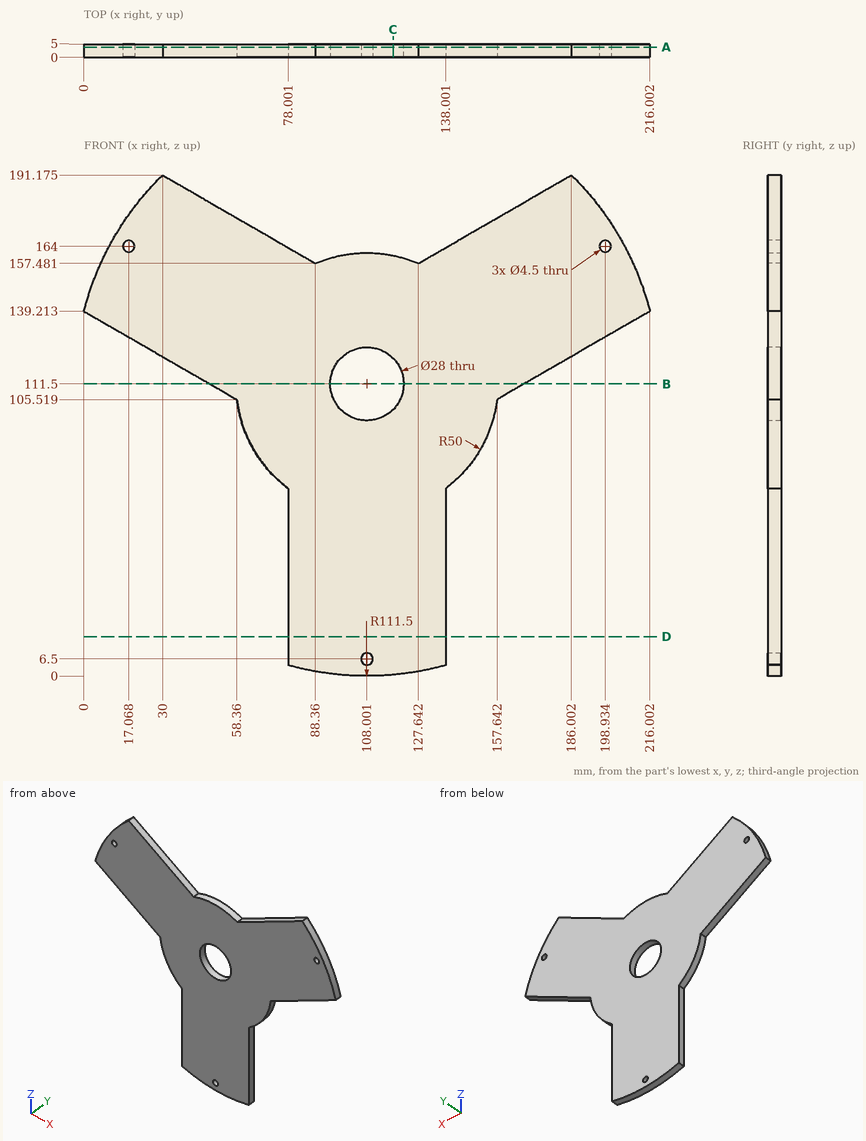
Geometry check sheet. Reference: drawing and pictorial views, mm from the part's lowest x, y, z. Round coordinates to 2 decimals unless told otherwise and drop trailing zeros. Loops run counter-clockwise (first coordinate to the right, second up) from the corner with the lowest first, then second, coordinate; pieces in that order, holes last. Notation, with made-up numbers: (36.25, -11.75) - (54.25, -11.75) arc R9 cw to (54.25, -1.75) - close; hole circle Ø9 at (-20.5, -28). An arc over 180 degrees is marked (long way). One line per question, with ' | ' between items. Start each with the question number.
1. Cross-section at D-D on z = 15. Record the cut outline in (x, y), then the cut area to 3 significant figures.
2. Cross-section at A-A on y = 3.85. State how many separate pieces and enclosed holes the cut face has, then the cut area to 3 significant figures.
3. Cross-section at B-B on z = 111.5. Record the cut outline in (x, y), then the cut area to 3 significant figures.
4. Scan lines: line 1 (X direction, y = 3.9, z = 164) (1 decimal); line 2 (X direction, y = 3.45, z = 52.5); line 3 (X direction, y = 3.6, z = 171) (1 decimal). Record each from-to range of solid material in increasing order. Write a range as [from, to].
5. Cross-section at C-C on x = 118. Record the cut outline in (y, z), then the cut area to 3 significant figures.
6. Depth check by flat-ended pin: pin 1 (2 mm diameter, centred on y = 1, z = 165, fed in from +X); pin 2 (3.5 mm diameter, centred on x = 17.07, z = 164, fed in from +Y); pin 3 (2 mm diameter, centred on y = 1.5, z = 27.5, fed in from -X). Enter the tip coordinate at first touch or a pass-through.
Taken from the geometry:
1) outline: (78, 0) - (138, 0) - (138, 5) - (78, 5) - close | area: 300 mm²
2) separate pieces: 1 | enclosed holes: 4 | area: 18,600 mm²
3) outline: (48, 0) - (94, 0) - (94, 5) - (48, 5) - close; (122, 0) - (168, 0) - (168, 5) - (122, 5) - close | area: 460 mm²
4) line 1: [9.6, 14.8], [19.3, 77.1], [138.9, 196.7], [201.2, 206.4] | line 2: [78, 138] | line 3: [13.7, 64.9], [151.1, 202.3]
5) outline: (0, 0.45) - (5, 0.45) - (5, 101.7) - (0, 101.7) - close; (0, 121.3) - (5, 121.3) - (5, 160.49) - (0, 160.49) - close | area: 702 mm²
6) pin 1: x = 206.37 | pin 2: through | pin 3: x = 78
